Answer from the drawing. Dimensions are ordinates in mm from the lowest x, y and z of the part. A direction names the side the tool comes from. Round coordinates to 2 decimals unless told otherwise and drop trailing zeros. Order: outer loops, then holes, each group sorted by start corner. A loop starts at its lowest first (then second) coordinate and runs counter-clockwise, first axis right, second up.
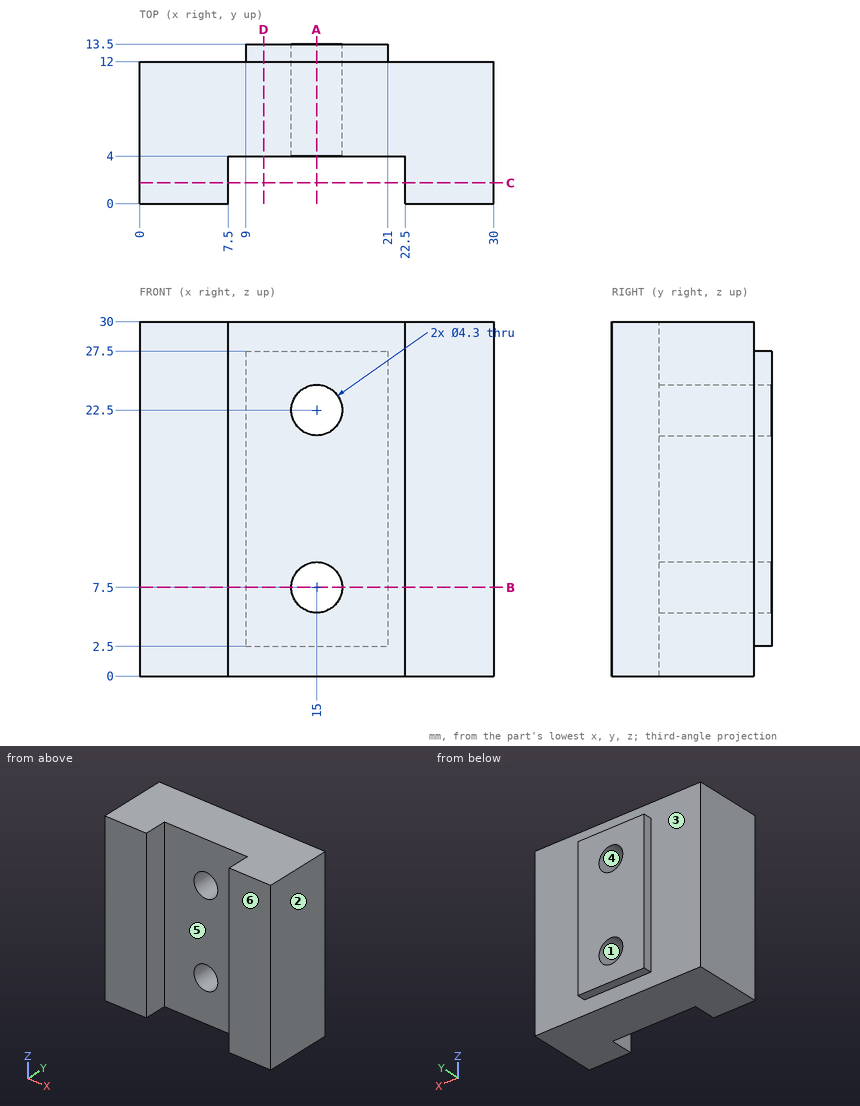
Q1. For a pull along X with two mould halves and no side action, classify the marked faces 1, 2, 3 and 4 as released by +X, released by -X, zero draft, split by the parting line, or undercut.
Outcome:
face 1: undercut
face 2: released by +X
face 3: zero draft
face 4: undercut
Q2. A cutting plane is placed at B-B, the plane z = 7.5. Give the vertices of the cut face in (x, y).
Outcome:
outline: (0, 0) - (7.5, 0) - (7.5, 4) - (12.85, 4) - (12.85, 13.5) - (9, 13.5) - (9, 12) - (0, 12) - close; (17.15, 4) - (22.5, 4) - (22.5, 0) - (30, 0) - (30, 12) - (21, 12) - (21, 13.5) - (17.15, 13.5) - close
Q3. For the marked faces 5 and 6, determine the directions among +Z, -Z, +X, -X, +Y, -Y from which every point of the face is accessible in a straight line to the end or side of a thin tool.
Outcome:
face 5: +Z, -Z, -Y
face 6: +Z, -Z, +X, -X, -Y
Q4. Straight lines are drawn through the part: probe 1 along X at (y, z) = (8.75, 7.5); probe 2 along Y at (x, z) = (3, 12.25); probe 3 along X at (y, z) = (2.25, 26). For each, find the intervals that lie inside material, in ascending order.
Outcome:
probe 1: x = 0 to 12.85, 17.15 to 30
probe 2: y = 0 to 12
probe 3: x = 0 to 7.5, 22.5 to 30
Q5. A cutting plane is placed at D-D, the plane x = 10.5. Give the vertices of the cut face in (y, z).
Outcome:
outline: (4, 0) - (12, 0) - (12, 2.5) - (13.5, 2.5) - (13.5, 27.5) - (12, 27.5) - (12, 30) - (4, 30) - close
Q6. Flat-ended cylindrical pins translate along their axes: pin 1 (1.2 mm diameter, centred on x = 14, y = 13, fed in from -Z); pin 2 (2 mm diameter, centred on x = 15, z = 15, fed in from -Y); pin 3 (3.5 mm diameter, centred on x = 15, z = 22.5, fed in from -Y); pin 4 (3 mm diameter, centred on x = 5, z = 25, fed in from +Y). Find the tip coordinate at first contact, or state that the pin passes through.
Outcome:
pin 1: stops at z = 2.5
pin 2: stops at y = 4
pin 3: passes through
pin 4: stops at y = 12
Q7. A cutting plane is placed at A-A, the plane x = 15. Give the vertices of the cut face in (y, z).
Outcome:
outline: (4, 0) - (12, 0) - (12, 2.5) - (13.5, 2.5) - (13.5, 5.35) - (4, 5.35) - close; (4, 9.65) - (13.5, 9.65) - (13.5, 20.35) - (4, 20.35) - close; (4, 24.65) - (13.5, 24.65) - (13.5, 27.5) - (12, 27.5) - (12, 30) - (4, 30) - close
Q8. A cutting plane is placed at C-C, the plane y = 1.75. Give the vertices of the cut face in (x, z), plus the area to 3 significant figures.
Outcome:
outline: (0, 0) - (7.5, 0) - (7.5, 30) - (0, 30) - close; (22.5, 0) - (30, 0) - (30, 30) - (22.5, 30) - close
area: 450 mm2
